from build123d import *

# Parameters (mm, degrees)
SKETCH1_W           = 25.1
SKETCH1_H           = 25.1
BOSS_EXTRUDE1_DEPTH = 32.85
SKETCH2_W           = 27
SKETCH2_H           = 27
BOSS_EXTRUDE2_DEPTH = 4
FILLET1_R           = 1
SKETCH3_R           = 1.415831881
SKETCH3_W           = 1.309672559
SKETCH3_H           = 7.543446756
SKETCH3_W_2         = 1.023845508
SKETCH3_H_2         = 7.18639052
CUT_EXTRUDE1_DEPTH  = 24


with BuildPart() as part:
    # Sketch1 → Boss-Extrude1 (new body)
    with BuildSketch(Plane.XY):
        Rectangle(SKETCH1_W, SKETCH1_H)
    extrude(amount=BOSS_EXTRUDE1_DEPTH)

    # Sketch2 → Boss-Extrude2 (add)
    with BuildSketch(Plane(origin=(0, 0, 0), x_dir=(-1, 0, 0), z_dir=(0, 0, -1))):
        Rectangle(SKETCH2_W, SKETCH2_H)
    extrude(amount=BOSS_EXTRUDE2_DEPTH)

    # Fillet1
    fillet1_edges = [part.edges().sort_by_distance(p)[0] for p in [
        (-13.5, 0, -4),
        (0, 13.5, -4),
        (13.5, 0, -4),
        (0, -13.5, -4),
    ]]
    fillet(fillet1_edges, radius=FILLET1_R)

    # Sketch3 → Cut-Extrude1 (cut)
    with BuildSketch(Plane(origin=(0, 0, -4), x_dir=(-1, 0, 0), z_dir=(0, 0, -1))):
        with Locations((0, -5.370956585)):
            Circle(SKETCH3_R)
        with Locations((-6.845163721, 5.728276622)):
            Rectangle(SKETCH3_W, SKETCH3_H)
        with Locations((6.988077246, 5.90680474)):
            Rectangle(SKETCH3_W_2, SKETCH3_H_2)
    extrude(amount=-CUT_EXTRUDE1_DEPTH, mode=Mode.SUBTRACT)


solid = part.part
Work out the finished part from the listing and answer in its coordinate system (mm). A direction names the side the tool comes from. Give positions to 0.01 mm unless a question says otherwise; leave off trailing zeros. Write each loop counter-clockwise with the first axis right and the second up, starting at its lowest first coordinate (ties: lowest second). Pieces come first, ordered by that corner, then holes.
Q1. The part is cut by section C-C on z = 2. Give the vertices of the cut face in (x, y).
Answer:
outline: (-12.55, -12.55) - (12.55, -12.55) - (12.55, 12.55) - (-12.55, 12.55) - close; hole (-7.5, 2.31) - (-6.48, 2.31) - (-6.48, 9.5) - (-7.5, 9.5) - close; hole circle Ø2.83 at (0, -5.37); hole (6.19, 1.96) - (7.5, 1.96) - (7.5, 9.5) - (6.19, 9.5) - close
Q2. The part is cut by section B-B on x = 0. Give the vertices of the cut face in (y, z), and give its area (3 significant figures).
Answer:
outline: (-13.5, -3) arc R1 ccw to (-12.5, -4) - (-6.79, -4) - (-6.79, 20) - (-3.96, 20) - (-3.96, -4) - (12.5, -4) arc R1 ccw to (13.5, -3) - (13.5, 0) - (12.55, 0) - (12.55, 32.85) - (-12.55, 32.85) - (-12.55, 0) - (-13.5, 0) - close
area: 864 mm2
Q3. For a pull along X with two mould halves and no side action, classify faces 1 (the face through (0, -12.55, 16)), 2 (the face through (7, 6, 20)), 3 (the face through (-13.5, 0, -1)) as released by +X, released by -X, zero draft, split by the parting line, or undercut.
Answer:
face 1: zero draft
face 2: undercut
face 3: released by -X
Q4. A tool of negligible diameter and unlimited length cuts with its end or side. For faces 4 (the face through (-0.189, 13.215, -3.699)), 5 (the face through (-7, 2.314, 8)), from which of +Z, -Z, +X, -X, +Y, -Y can it reach the whole face along a straight path? Write none if from no direction.
Answer:
face 4: -Z, +X, -X, +Y
face 5: -Z
Q5. Straight lines are drawn through the part: L1, parallel to X at y = 5.5, z = 5.5; L2, parallel to Y at x = 0, z = 15; L3, parallel to X at y = 12.5, z = 25.5. For each, find the intervals that lie inside material, in ascending order.
Answer:
L1: x = -12.55 to -7.5, -6.48 to 6.19, 7.5 to 12.55
L2: y = -12.55 to -6.79, -3.96 to 12.55
L3: x = -12.55 to 12.55
Q6. The part is cut by section D-D on y = -10.25. Give the vertices of the cut face in (x, z).
Answer:
outline: (-13.5, -3) arc R1 ccw to (-12.5, -4) - (12.5, -4) arc R1 ccw to (13.5, -3) - (13.5, 0) - (12.55, 0) - (12.55, 32.85) - (-12.55, 32.85) - (-12.55, 0) - (-13.5, 0) - close
Q7. The part is cut by section A-A on y = 5.75. Give the vertices of the cut face in (x, z).
Answer:
outline: (-13.5, -3) arc R1 ccw to (-12.5, -4) - (-7.5, -4) - (-7.5, 20) - (-6.48, 20) - (-6.48, -4) - (6.19, -4) - (6.19, 20) - (7.5, 20) - (7.5, -4) - (12.5, -4) arc R1 ccw to (13.5, -3) - (13.5, 0) - (12.55, 0) - (12.55, 32.85) - (-12.55, 32.85) - (-12.55, 0) - (-13.5, 0) - close
Q8. Given pin 1 (1.1 mm diameter, centred on x = -7, z = 2, fed in from +Y); pin 2 (1.5 mm diameter, centred on y = 2, z = 22.5, fed in from -X); pin 3 (10 mm diameter, centred on y = -0.5, z = 9.5, fed in from +X); pin 4 (3 mm diameter, centred on x = -0.5, y = -5.5, fed in from -Z), each flat-ended and moving along its own axis, determine where each tip first touches the part or whether it passes through.
Answer:
pin 1: stops at y = 12.55
pin 2: stops at x = -12.55
pin 3: stops at x = 12.55
pin 4: stops at z = -4
